Autodesk Inventor part; units mm, degrees
ref_plane "YZ Plane" through (0, 0, 0) normal (1, 0, 0) x (0, 1, 0)
ref_plane "XZ Plane" through (0, 0, 0) normal (0, 1, 0) x (-1, 0, 0)
ref_plane "XY Plane" through (0, 0, 0) normal (0, 0, 1) x (1, 0, 0)
sketch "Sketch1" plane through (0, 0, 0) normal (0, 1, 0) x (-1, 0, 0)
  line L0 (0, 0) -> (25.4, 0)
  line L1 (25.4, 0) -> (25.4, 25.4)
  line L2 (25.4, 25.4) -> (0, 25.4)
  line L3 (0, 25.4) -> (0, 0)
  dimension "d0" = 25.4
  dimension "d1" = 25.4
extrude "Extrusion1" add sketch "Sketch1" along normal blind 6.35
sketch "Sketch2" plane through (0, 6.35, 0) normal (0, 1, 0) x (1, 0, 0)
  line L0 (-25.4, 0) -> (-25.4, -25.4)
  line L1 (0, 0) -> (-25.4, 0)
  point P0 (-12.7, -12.7)
  point P1 (-25.4, -12.7)
  point P2 (-12.7, 0)
hole "Hole1" at (-12.7, 6.35, 12.7) direction (0, -1, 0) diameter 4.1402 end through all
properties part number ".25inAlluminumspacer-ver1-1111-2018"
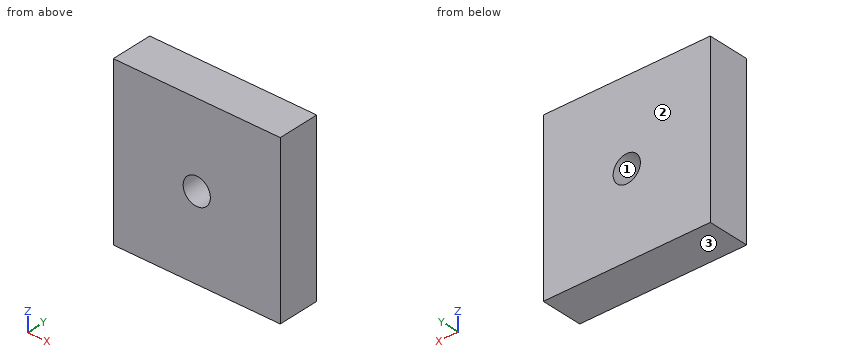
Geometry check sheet. Reference: the model listing, model coordinates, mm. Face numbers are marked on the shaded views. Give positions to 0.01 mm unless a question says otherwise; leave off trailing zeros. Write each loop counter-clockwise with the first axis right and the second up, starting at its lowest first coordinate (ties: lowest second). Pieces come first, ordered by that corner, then holes.
1) Section check C-C, the plane y = 3.5. Record the boundary of the cut face in (x, z), and give its area (3 significant figures).
2) Material ranges on L1, parallel to Z at x = -12.7, y = 3.5; L2, parallel to X at y = 4, z = 12.7; L3, parallel to X at y = 2, z = 11.5, recorded low to high.
3) Section check B-B, the plane z = 12.7. Record the boundary of the cut face in (x, y).
4) Section check A-A, the plane x = -12.7. Record the boundary of the cut face in (y, z), and give its area (3 significant figures).
5) Release check for a two-part mould opening along Z. For the marked faces 1, 2 and 3 record: pulls with the +Z half, pulls with the -Z half, needs draft (parallel to the pull), parting line crosses it, or undercut.
Computed:
1. outline: (-25.4, 0) - (0, 0) - (0, 25.4) - (-25.4, 25.4) - close; hole circle Ø4.14 at (-12.7, 12.7)
1. area: 632 mm2
2. L1: z = 0 to 10.63, 14.77 to 25.4
2. L2: x = -25.4 to -14.77, -10.63 to 0
2. L3: x = -25.4 to -14.39, -11.01 to 0
3. outline: (-25.4, 0) - (-14.77, 0) - (-14.77, 6.35) - (-25.4, 6.35) - close; (-10.63, 0) - (0, 0) - (0, 6.35) - (-10.63, 6.35) - close
4. outline: (0, 0) - (6.35, 0) - (6.35, 10.63) - (0, 10.63) - close; (0, 14.77) - (6.35, 14.77) - (6.35, 25.4) - (0, 25.4) - close
4. area: 135 mm2
5. face 1: undercut
5. face 2: needs draft
5. face 3: pulls with the -Z half
